Can you work these out from the model? Positions are in its coordinate system, mm. A direction names the side the tool comes from. Round coordinates to 2 decimals unless told otherwise and drop trailing zeros. Loops run counter-clockwise (first coordinate to the right, second up) from the corner with the lowest first, then second, coordinate; pieces in that order, holes last. Notation, with made-up numbers: M 23.5,0 L 61.5,0 A22 cw 61.5,8 Z; hole C 5,7 d5. An arc over 180 degrees is marked long. Answer as CSV lines item,"result".
Autodesk Inventor part; units mm, degrees
ref_plane "Start Plane" through (0, 0, 8.391) normal (0, 0, 1) x (1, 0, 0)
ref_plane "End Plane" through (0, 0, 60) normal (0, 0, 1) x (1, 0, 0)
ref_plane "Work Plane4" through (-6.5, -25.0184, 42.0413) normal (0, 0.9318, -0.363) x (0, 0.363, 0.9318)
ref_plane "Start Plane" through (0, 0, 8.391) normal (0, 0, 1) x (1, 0, 0)
ref_plane "End Plane" through (0, 0, 60) normal (0, 0, 1) x (1, 0, 0)
sketch "Sketch" plane through (0, 0, 0) normal (0, 0, 1) x (1, 0, 0)
  line L0 (-10, -7) -> (-10, 7)
  line L1 (-7, 10) -> (7, 10)
  line L2 (10, 7) -> (10, -7)
  line L3 (7, -10) -> (-7, -10)
  arc A0 (-10, -7) -> (-7, -10) centre (-7, -7) ccw
  arc A1 (-7, 10) -> (-10, 7) centre (-7, 7) ccw
  arc A2 (10, 7) -> (7, 10) centre (7, 7) ccw
  arc A3 (7, -10) -> (10, -7) centre (7, -7) ccw
  arc A4 (-7, 8) -> (-8, 7) centre (-7, 7) ccw
  line L4 (-7, 8) -> (7, 8)
  arc A5 (8, 7) -> (7, 8) centre (7, 7) ccw
  line L5 (8, 7) -> (8, -7)
  arc A6 (7, -8) -> (8, -7) centre (7, -7) ccw
  line L6 (7, -8) -> (-7, -8)
  arc A7 (-8, -7) -> (-7, -8) centre (-7, -7) ccw
  line L7 (-8, -7) -> (-8, 7)
  line L8 (0, 14.8698) -> (0, -14.8698) construction
  line L9 (-14.8698, 0) -> (14.8698, 0) construction
  dimension "d7" = 3
  dimension "d10" = 20
  dimension "d11" = 20
  dimension "d12" = 2
  dimension "d15" = 10
  dimension "d16" = 10
extrude "Body" add sketch "Sketch" along normal up to surface (51.609 mm away) from surface at 8.391
sketch "Sketch3" plane through (0, 0, 0) normal (0, 0, 1) x (1, 0, 0)
  line L0 (0, 0) -> (10, 0)
ref_plane "Work Plane3" through (0, 0, 0) normal (0, -1, 0) x (1, 0, 0)
sketch "Sketch4" plane through (0, 0, 0) normal (0, -1, 0) x (1, 0, 0)
  line L0 (-2, 8.391) -> (12, 8.391)
  line L1 (-2, 60) -> (12, 60)
  dimension "d18" = 51.609
sketch "Sketch5" plane through (-7, -10, 60) normal (0, 0, 1) x (1, 0, 0)
  line L0 (14, 18) -> (0, 18)
  arc A0 (15, 17) -> (14, 18) centre (14, 17) ccw
  line L1 (15, 3) -> (15, 17)
  arc A1 (14, 2) -> (15, 3) centre (14, 3) ccw
  line L2 (0, 2) -> (14, 2)
  arc A2 (-1, 3) -> (0, 2) centre (0, 3) ccw
  line L3 (-1, 17) -> (-1, 3)
  arc A3 (0, 18) -> (-1, 17) centre (0, 17) ccw
  line L4 (-3, 3) -> (-3, 17)
  arc A4 (-3, 3) -> (0, 0) centre (0, 3) ccw
  line L5 (14, 0) -> (0, 0)
  arc A5 (14, 0) -> (17, 3) centre (14, 3) ccw
  line L6 (17, 17) -> (17, 3)
  arc A6 (17, 17) -> (14, 20) centre (14, 17) ccw
  line L7 (0, 20) -> (14, 20)
  arc A7 (0, 20) -> (-3, 17) centre (0, 17) ccw
  point P0 (7, 10)
ref_plane "Work Plane4" through (-6.5, -25.0184, 42.0413) normal (0, 0.9318, -0.363) x (0, 0.363, 0.9318)
ref_plane "Work Plane5" through (-6.5, -27.0573, 38.5716) normal (0, 0.8829, -0.4695) x (0, 0.4695, 0.8829)
ref_plane "Work Plane7" through (-6.5, -28.4333, 41.6034) normal (0, 0.8611, -0.5085) x (0, 0.5085, 0.8611)
ref_plane "Work Plane8" through (-6.5, -28.4333, 41.6034) normal (0, 0.8611, -0.5085) x (0, 0.5085, 0.8611)
extrude "Extrusion2" add sketch "Sketch5" along normal up to surface surface through (-6.5, -28.4333, 41.6034) normal (0, 0.8611, -0.5085)
ref_plane "Work Plane6" through (75, 8.6301, 8.6325) normal (0, -0.1736, -0.9848) x (1, 0, 0)
split "Split1" plane through (75, 8.6301, 8.6325) removes the side toward (0, -0.1736, -0.9848)
equation "\"d7\" = G_IR"
equation "\"d10\" = G_H"
equation "\"d11\" = G_W"
equation "\"d12\" = G_T"
equation "\"d15\" = 0.5 * d10"
equation "\"d16\" = 0.5 * d11"
equation "\"d3\" = G_L"
equation "\"G_W\" = 20"
equation "\"G_H\" = 20"
equation "\"G_T\" = 2"
equation "\"G_IR\" = 3"
equation "\"G_L\" = 98.29424"
equation "\"G_OFFSET_START\" = -8.391"
equation "\"G_OFFSET_END\" = 0"
equation "\"d13\" = -G_OFFSET_START"
properties part number "ISO 12633-2 - 20x20x2 - 98,29" material "Steel, Mild"
Item 1: If we section it at B-B on z = 61: Write out the boundary of the cut face in (x, y), then the cut area to 3 significant figures.
Output:
outline,"M -10,-7 A3 ccw -7,-10 L 7,-10 A3 ccw 10,-7 L 10,7 A3 ccw 7,10 L -7,10 A3 ccw -10,7 Z; hole M -8,-7 A1 ccw -7,-8 L 7,-8 A1 ccw 8,-7 L 8,7 A1 ccw 7,8 L -7,8 A1 ccw -8,7 Z"
area,"137 mm2"
Item 2: If we section it at D-D on y = 0: Write out the boundary of the cut face in (x, z), then the cut area to 3 significant figures.
Output:
outline,"M -10,10.15 L -8,10.15 L -8,89.75 L -10,89.75 Z; M 8,10.15 L 10,10.15 L 10,89.75 L 8,89.75 Z"
area,"318 mm2"
Item 3: If we section it at C-C on y = 4.75: Write out the boundary of the cut face in (x, z), then the cut area to 3 significant figures.
Output:
outline,"M -10,9.32 L -8,9.32 L -8,97.8 L -10,97.8 Z; M 8,9.32 L 10,9.32 L 10,97.8 L 8,97.8 Z"
area,"354 mm2"
Item 4: If I drill on line 1 along X through (y, z) = (4.25, 84.5); line 2 along Y through (x, z) = (0.25, 101.5), over which ranges is the centre line in solid material (lowest first)? Write a range as from..to.
Output:
line 1,"x = -10..-8, 8..10"
line 2,"y = 8..10"
Item 5: We'd pull the mould along X, two halves only. Please class faces 1 (the face through (-9.1, -9.14, 44.18)), 2 (the face through (10, 0, 44)), 3 (the face through (-8, 0, 44)): released by +X, released by -X, zero draft, split by the parting line, or undercut.
Output:
face 1,"released by -X"
face 2,"released by +X"
face 3,"undercut"
Item 6: On a 3-axis mill with a long thin cutter (end or side, diameter ignored), from which of +Z, -Z, +X, -X, +Y, -Y can I reach the whole of each face in a straight line? I mean faces 4 (the face through (0, -10, 42)), 5 (the face through (0, -8, 43)). Say none if no direction works.
Output:
face 4,"+Z, -Z, +X, -X, -Y"
face 5,"+Z, -Z"
